Source: CAD feature listing. Evaluate the final solid. Frame: model axes, mm. A direction names the side the tool comes from. Coordinates: 2 decimals unless noted, no trailing zeros. Loops run counter-clockwise (first coordinate to the right, second up) from the corner with the lowest first, then second, coordinate; pieces in that order, holes last. Notation, with made-up numbers: (-13, 62.25) - (22, 62.25) arc R22 ccw to (22, 99.25) - close; hole circle Ø7 at (-16, 81). An arc over 180 degrees is marked (long way). Write item = value, one per line. Start each with the question number.
from build123d import *

# Parameters (mm, degrees)
BOSS_EXTRUDE3_DEPTH     = 8.75
CUT_EXTRUDE1_DEPTH      = 30.433335283
CUT_EXTRUDE1_DEPTH_BACK = 30.433335283
SKETCH2_R               = 6.5
CUT_EXTRUDE2_DEPTH      = 30.248560932
CUT_EXTRUDE2_DEPTH_BACK = 30.248560932
SKETCH3_R               = 6.5


with BuildPart() as part:
    # Sketch1 → Boss-Extrude3 (new, symmetric)
    with BuildSketch(Plane(origin=(0, 0, 0), x_dir=(1, 0, 0), z_dir=(0, 1, 0))):
        with BuildLine():
            Line((14.3, -12), (0, -12))
            ThreePointArc((0, -12), (-8.929217577, -8.016799453), (-11.930624431, 1.288487755))
            Line((-11.930624431, 1.288487755), (-11.256544629, 7.530062747))
            ThreePointArc((-11.256544629, 7.530062747), (-12.453785005, 9.017212868), (-10.966634884, 10.214453244))
            Line((-10.966634884, 10.214453244), (-10.805573915, 11.705781297))
            ThreePointArc((-10.805573915, 11.705781297), (-11.574951792, 13.180943013), (-9.917441597, 13.324833112))
            Line((-9.917441597, 13.324833112), (-7.001026651, 9.680635575))
            Line((-7.001026651, 9.680635575), (-8.989464056, 9.895383534))
            Line((-8.989464056, 9.895383534), (-7.217023351, 7.680635575))
            Line((-7.217023351, 7.680635575), (-9.205460756, 7.895383534))
            Line((-9.205460756, 7.895383534), (-7.433020052, 5.680635575))
            Line((-7.433020052, 5.680635575), (-9.421457457, 5.895383534))
            Line((-9.421457457, 5.895383534), (-7.649016752, 3.680635575))
            Line((-7.649016752, 3.680635575), (-9.637454157, 3.895383534))
            Line((-9.637454157, 3.895383534), (-9.942187026, 1.073739796))
            ThreePointArc((-9.942187026, 1.073739796), (-7.441014647, -6.680666211), (0, -10))
            Line((0, -10), (3, -10))
            ThreePointArc((3, -10), (3.640312424, -9.77539053), (4, -9.2))
            ThreePointArc((4, -9.2), (4.359687576, -8.62460947), (5, -8.4))
            Line((5, -8.4), (6.5, -8.4))
            ThreePointArc((6.5, -8.4), (6.853553391, -8.253553391), (7, -7.9))
            Line((7, -7.9), (7, -7.8))
            ThreePointArc((7, -7.8), (9.8, -5), (12.6, -7.8))
            ThreePointArc((12.6, -7.8), (13.097918472, -9.002081528), (14.3, -9.5))
            ThreePointArc((14.3, -9.5), (21.749280739, -2.870756267), (16.029735438, 5.297808939))
            ThreePointArc((16.029735438, 5.297808939), (12.818459255, 4.77966532), (10.914126957, 2.142567288))
            ThreePointArc((10.914126957, 2.142567288), (7.604027352, 0.100940338), (5.562400402, 3.411039943))
            ThreePointArc((5.562400402, 3.411039943), (5.044256782, 6.622316125), (2.407158751, 8.526648423))
            Line((2.407158751, 8.526648423), (-6.836732572, 10.717646644))
            Line((-6.836732572, 10.717646644), (-8.692757073, 13.726828103))
            Line((-8.692757073, 13.726828103), (16.606313917, 7.730411919))
            ThreePointArc((16.606313917, 7.730411919), (24.232374318, -3.161008357), (14.3, -12))
        make_face()
    extrude(amount=BOSS_EXTRUDE3_DEPTH, both=True)

    # Sketch2 → Cut-Extrude1 (cut, two sides: drawn at the far end of the back side and taken through both)
    with BuildSketch(Plane(origin=(-0.037875914, 0, 0.324026741), x_dir=(0.9932374318152281, 0, 0.11610083566060259), z_dir=(-0.11610083566060259, 0, 0.9932374318152281)).offset(-CUT_EXTRUDE1_DEPTH_BACK)):
        with Locations((24.435496946, 0)):
            Circle(SKETCH2_R)
    extrude(amount=CUT_EXTRUDE1_DEPTH + CUT_EXTRUDE1_DEPTH_BACK, mode=Mode.SUBTRACT)

    # Sketch3 → Cut-Extrude2 (cut, two sides: drawn at the far end of the back side and taken through both)
    with BuildSketch(Plane(origin=(0, 0, 0), x_dir=(-0.7441014647171004, 0, 0.6680666210834559), z_dir=(-0.6680666210834559, 0, -0.7441014647171004)).offset(-CUT_EXTRUDE2_DEPTH_BACK)):
        with Locations((12, 0)):
            Circle(SKETCH3_R)
    extrude(amount=CUT_EXTRUDE2_DEPTH + CUT_EXTRUDE2_DEPTH_BACK, mode=Mode.SUBTRACT)


solid = part.part
Item 1: Material intervals for L1, parallel to X at y = 7.5, z = -3.25; L2, parallel to X at y = 6.75, z = -4.75; L3, parallel to Z at x = 16, y = 7.5, sorted ascending. Write a range as [from, to].
Item 2: Cut plane C-C (y = 3). State how many separate pieces and enclosed holes the cut face has, then the cut area to 3 significant figures.
Item 3: Cut plane B-B (z = -12.7). Return the cut outline in (x, y).
Item 4: Cut plane A-A (x = 9.8). Return the cut outline in (y, z), then the cut area to 3 significant figures.
Item 5: Reachability of faces 4 (the flat face through (-11.523, 0.123, -5.059)), 5 (the flat face through (3.78, 0.12, -10.77)), 6 (the cylindrical face through (-7.52, -7.32, 6.59)) from +Z, -Z, +X, -X, +Y, -Y: full face, straight path, thin tool, end or side. Return the list, or none.
Item 6: First-contact query: pin 1 (2.5 mm diameter, centred on x = 1.5, y = 4, fed in from -Z); pin 2 (5 mm diameter, centred on x = 6.5, y = 0.5, fed in from -Z); pin 3 (10 mm diameter, centred on y = 6.5, z = -7, fed in from +X); pin 4 (4 mm diameter, centred on x = -4, z = -5, fed in from -Y). Flat tips, straight axial feed; report the tip coordinate or a pass-through.
Item 7: Draft query along Y for faces 1 (the flat face through (6, -8.75, -4)), 2 (the cylindrical face through (22.987, -6.375, 2.883)), 3 (the flat face through (-2.15, 0.123, -9.607)). Return one class per face: released by +Y, released by -Y, zero draft, split by the parting line, or undercut.
Responses:
q1.L1 = [-11.72, -9.71], [5.53, 11.35], [19.66, 22.81]
q1.L2 = [-11.56, -8.5], [5.66, 12.77], [17.57, 21.68]
q1.L3 = [-7.87, -5.3], [9.3, 11.85]
q2.separate_pieces = 3
q2.enclosed_holes = 0
q2.area = 212 mm2
q3.outline = (-11.7, -8.75) - (-9.42, -8.75) - (-9.42, 8.75) - (-11.7, 8.75) - close; (-8.06, -8.75) - (-4.36, -8.75) - (-4.36, 8.75) - (-8.06, 8.75) - close
q4.outline = (-8.75, -9.34) - (8.75, -9.34) - (8.75, -0.51) - (-8.75, -0.51) - close; (-8.75, 5) - (8.75, 5) - (8.75, 12) - (-8.75, 12) - close
q4.area = 277 mm2
q5.face_4 = -X, +Y, -Y
q5.face_5 = -Z, +X, +Y, -Y
q5.face_6 = +Y, -Y
q6.pin_1 = -11.61
q6.pin_2 = -10.72
q6.pin_3 = 23.47
q6.pin_4 = through
q7.face_1 = released by -Y
q7.face_2 = undercut
q7.face_3 = zero draft
